```python
from build123d import *

# Parameters (mm, degrees)
BOSS_EXTRUDE1_DEPTH = 1
FILLET1_R           = 10
BOSS_EXTRUDE2_START = 16
BOSS_EXTRUDE2_DEPTH = 16
BOSS_EXTRUDE3_DEPTH = 5.5


with BuildPart() as part:
    # Sketch1 → Boss-Extrude1 (new body)
    with BuildSketch(Plane.XY):
        Polygon((-59.5, 15), (59.5, 15), (59.5, 5.5), (64.5, 5.5), (64.5, -44.3), (-64.5, -44.3), (-64.5, 5.5), (-59.5, 5.5), align=None)
    extrude(amount=BOSS_EXTRUDE1_DEPTH)

    # Fillet1
    fillet1_edges = [part.edges().sort_by_distance(p)[0] for p in [
        (64.5, -44.3, 0.5),
        (-64.5, -44.3, 0.5),
    ]]
    fillet(fillet1_edges, radius=FILLET1_R)

    # Sketch2 → Boss-Extrude2 (add)
    with BuildSketch(Plane.XY.offset(1).offset(BOSS_EXTRUDE2_START)):
        with BuildLine():
            Line((59.5, 5.5), (59.5, 15))
            Line((59.5, 15), (-59.5, 15))
            Line((-59.5, 15), (-59.5, 5.5))
            Line((-59.5, 5.5), (-64.5, 5.5))
            Line((-64.5, 5.5), (-64.5, -34.3))
            ThreePointArc((-64.5, -34.3), (-61.571067812, -41.371067812), (-54.5, -44.3))
            Line((-54.5, -44.3), (54.5, -44.3))
            ThreePointArc((54.5, -44.3), (61.571067812, -41.371067812), (64.5, -34.3))
            Line((64.5, -34.3), (64.5, 5.5))
            Line((64.5, 5.5), (59.5, 5.5))
        make_face()
        with BuildLine():
            Line((-54.5, -42.3), (54.5, -42.3))
            ThreePointArc((54.5, -42.3), (60.156854249, -39.956854249), (62.5, -34.3))
            Line((62.5, -34.3), (62.5, 3.5))
            Line((62.5, 3.5), (57.5, 3.5))
            Line((57.5, 3.5), (57.5, 13))
            Line((57.5, 13), (-57.5, 13))
            Line((-57.5, 13), (-57.5, 3.5))
            Line((-57.5, 3.5), (-62.5, 3.5))
            Line((-62.5, 3.5), (-62.5, -34.3))
            ThreePointArc((-62.5, -34.3), (-60.156854249, -39.956854249), (-54.5, -42.3))
        make_face(mode=Mode.SUBTRACT)
    extrude(amount=-BOSS_EXTRUDE2_DEPTH)

    # Sketch3 → Boss-Extrude3 (add)
    with BuildSketch(Plane.XY.offset(1)):
        Polygon((-20.877513704, 2), (21.122486296, 2), (21.122486296, 13), (57.5, 13), (57.5, 3.5), (62.5, 3.5), (62.5, 0), (-62.5, 0), (-62.5, 3.5), (-57.5, 3.5), (-57.5, 13), (-20.877513704, 13), align=None)
    extrude(amount=BOSS_EXTRUDE3_DEPTH)


solid = part.part
```
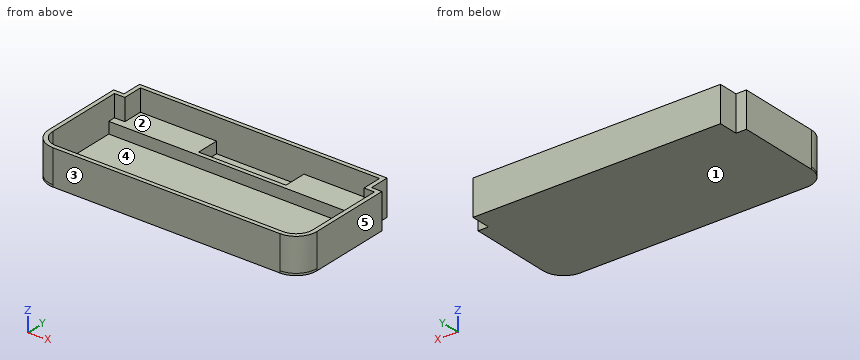
Verification items for the finished model (mm, model axes). Face numbers are marked on the shaded views. A direction names the side the tool comes from. Give positions to 0.01 mm unless a question says otherwise; leave off trailing zeros. Order: outer loops, then holes, each group sorted by start corner. A loop starts at its lowest first (then second) coordinate and runs counter-clockwise, first axis right, second up. Notation, with made-up numbers: M 67,13 L 116,13 A6 cw 116,24 Z; hole C 4,-38.5 d8. An arc over 180 degrees is marked long. Answer in a Markdown table with one row per item. Add a question column.
Item 1: Section check A-A, the plane z = 14. Enter the section's corners in (x, y).
Item 2: Section check C-C, the plane x = -37. Enter the section's corners in (y, z).
Item 3: Scan lines: probe 1 along Y at (x, z) = (-19.5, 2.25); probe 2 along X at (y, z) = (-2, 5.5); probe 3 along X at (y, z) = (12, 9.5). Record each from-to range of solid material in increasing order. Write a range as from..to.
Item 4: Tool access check on the marked faces 4 and 5. Record the directions out of +Z, -Z, +X, -X, +Y, -Y that give a thin tool (end or side, any length) a straight path to the whole face; none if there is none.
Item 5: Section check B-B, the plane y = -10.5. Enter the section's corners in (x, z), and give its area (3 significant figures).
Item 6: Mould release check, pull along Y, two halves, no side actions. Record for the marked faces 1, 2 and 3: released by +Y, released by -Y, zero draft, split by the parting line, or undercut.
Item 7: Section check D-D, the plane z = 4. Enter the section's corners in (x, y), and give its area (3 significant figures).
Item 8: Gauge pin test, flat ends, axial feed: pin 1 (8 mm diameter, centred on x = 28, y = 0, fed in from +Z); pin 2 (1.5 mm diameter, centred on x = -62, z = 11.5, fed in from +Y); pin 3 (4 mm diameter, centred on x = -60.5, z = 12.5, fed in from -Y). Record the tip position at first contact, or that the pin passes through.
Filled sheet:
| question | item | result |
|---|---|---|
| 1 | outline | M -64.5,-34.3 A10 ccw -54.5,-44.3 L 54.5,-44.3 A10 ccw 64.5,-34.3 L 64.5,5.5 L 59.5,5.5 L 59.5,15 L -59.5,15 L -59.5,5.5 L -64.5,5.5 Z; hole M -62.5,-34.3 A8 ccw -54.5,-42.3 L 54.5,-42.3 A8 ccw 62.5,-34.3 L 62.5,3.5 L 57.5,3.5 L 57.5,13 L -57.5,13 L -57.5,3.5 L -62.5,3.5 Z |
| 2 | outline | M -44.3,0 L 15,0 L 15,17 L 13,17 L 13,6.5 L 0,6.5 L 0,1 L -42.3,1 L -42.3,17 L -44.3,17 Z |
| 3 | probe 1 | y = -44.3..-42.3, 0..2, 13..15 |
| 3 | probe 2 | x = -64.5..-62.5, 62.5..64.5 |
| 3 | probe 3 | x = -59.5..-57.5, 57.5..59.5 |
| 4 | face 4 | +Z |
| 4 | face 5 | +Z, -Z, +X, +Y, -Y |
| 5 | outline | M -64.5,0 L 64.5,0 L 64.5,17 L 62.5,17 L 62.5,1 L -62.5,1 L -62.5,17 L -64.5,17 Z |
| 5 | area | 193 mm^2 |
| 6 | face 1 | zero draft |
| 6 | face 2 | undercut |
| 6 | face 3 | released by -Y |
| 7 | outline | M -64.5,-34.3 A10 ccw -54.5,-44.3 L 54.5,-44.3 A10 ccw 64.5,-34.3 L 64.5,5.5 L 59.5,5.5 L 59.5,15 L -59.5,15 L -59.5,5.5 L -64.5,5.5 Z; hole M -62.5,-34.3 A8 ccw -54.5,-42.3 L 54.5,-42.3 A8 ccw 62.5,-34.3 L 62.5,0 L -62.5,0 Z; hole M -20.88,2 L 21.12,2 L 21.12,13 L -20.88,13 Z |
| 7 | area | 1,790 mm^2 |
| 8 | pin 1 | stops at z = 6.5 |
| 8 | pin 2 | stops at y = 5.5 |
| 8 | pin 3 | stops at y = -43.47 |
